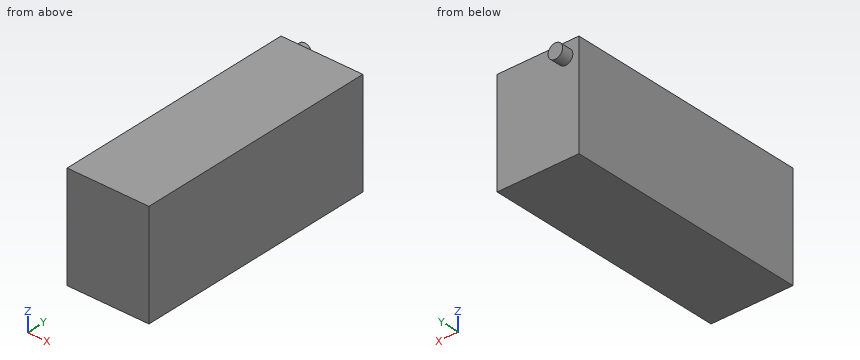
from build123d import *

# Parameters (mm, degrees)
SKETCH1_W             = 70
SKETCH1_H             = 210
LV_BATTRY_DEPTH       = 90
SKETCH2_R             = 6.25
CABLES_3X_14AWG_DEPTH = 10


with BuildPart() as part:
    # Sketch1 → LV Battry (new body)
    with BuildSketch(Plane.XY):
        with Locations((-86.457724765, 45.558894231)):
            Rectangle(SKETCH1_W, SKETCH1_H)
    extrude(amount=LV_BATTRY_DEPTH)

    # Sketch2 → Cables (3x 14AWG) (add)
    with BuildSketch(Plane(origin=(0, 150.558894231, 0), x_dir=(1, 0, 0), z_dir=(0, 1, 0))):
        with Locations(Location((-109.957724765, -78.5, 0), (0, 0, 90))):
            Circle(SKETCH2_R)
    extrude(amount=CABLES_3X_14AWG_DEPTH)


solid = part.part
Source: CAD feature listing. Evaluate the final solid. Frame: model axes, mm. Coordinates: 2 decimals unless noted, no trailing zeros. Loops run counter-clockwise (first coordinate to the right, second up) from the corner with the lowest first, then second, coordinate; pieces in that order, holes last. Notation, with made-up numbers: (84, 34) - (99, 34) arc R24 ccw to (99, 46) - close; hole circle Ø5 at (-31.5, -23). An arc over 180 degrees is marked (long way). One line per question, with ' | ' between items.
1) Section A-A, the plane z = 78.5. Return loops of the section in (x, y).
Report:
outline: (-121.46, -59.44) - (-51.46, -59.44) - (-51.46, 150.56) - (-103.71, 150.56) - (-103.71, 160.56) - (-116.21, 160.56) - (-116.21, 150.56) - (-121.46, 150.56) - close
2) First-contact query: P1, Ø1.5, axis at x = -73.5, z = 69, coming from the +Y side. Flat tip, straight axial feed; report the tip coordinate or a pass-through.
Report:
P1: stops at y = 150.56
3) Section B-B, the plane x = -89.5. Return loops of the section in (y, z).
Report:
outline: (-59.44, 0) - (150.56, 0) - (150.56, 90) - (-59.44, 90) - close
4) Section C-C, the plane z = 68. Return loops of the section in (x, y).
Report:
outline: (-121.46, -59.44) - (-51.46, -59.44) - (-51.46, 150.56) - (-121.46, 150.56) - close
5) Line query: line 1 along Y through (x, z) = (-97, 31). Output: solid intervals per line, ascending.
Report:
line 1: y = -59.44 to 150.56
